Input: part model. Units: mm. Frame: model coordinates. Coordinates: 2 decimals unless noted, no trailing zeros. Write each loop counter-clockwise with the first axis right and the second up, starting at its lowest first coordinate (ties: lowest second). Pieces come first, ordered by that corner, then holes.
from build123d import *

# Parameters (mm, degrees)
F0_W     = 7.9375
F0_H     = 12.7
F0_W_2   = 34.925
F1_DEPTH = 12.7
F3_D     = 4.7625
F5_DEPTH = 50.8


with BuildPart() as f1:
    # F0 (on Front) → F1 (new body, symmetric)
    with BuildSketch(Plane.XZ):
        with Locations((3.96875, -6.35)):
            Rectangle(F0_W, F0_H)
        with Locations((25.4, -6.35)):
            Rectangle(F0_W_2, F0_H)
        with Locations((46.83125, -6.35)):
            Rectangle(F0_W, F0_H)
        with Locations((3.96875, 6.35)):
            Rectangle(F0_W, F0_H)
        with Locations((25.4, 6.35)):
            Rectangle(F0_W_2, F0_H)
        with Locations((46.83125, 6.35)):
            Rectangle(F0_W, F0_H)
    extrude(amount=F1_DEPTH, both=True)

    # F3 (through all)
    with Locations(Plane.XZ.offset(12.7)):
        with Locations((7.9375, 0), (42.8625, 0)):
            Hole(F3_D / 2)

    # F4 (on face) → F5 (cut)
    with BuildSketch(Plane(origin=(0, 0, 0), x_dir=(0, -1, 0), z_dir=(-1, 0, 0))):
        with BuildLine():
            Line((12.7, -12.7), (12.7, 0))
            ThreePointArc((12.7, 0), (8.9802561211, -8.9802561211), (0, -12.7))
            Line((0, -12.7), (12.7, -12.7))
        make_face()
        with BuildLine():
            Line((-12.7, -12.7), (0, -12.7))
            ThreePointArc((0, -12.7), (-8.9802561211, -8.9802561211), (-12.7, 0))
            Line((-12.7, 0), (-12.7, -12.7))
        make_face()
        with BuildLine():
            ThreePointArc((-12.7, 0), (-8.9802561145, 8.9802561276), (1.86e-08, 12.7))
            Line((1.86e-08, 12.7), (-12.7, 12.7))
            Line((-12.7, 12.7), (-12.7, 0))
        make_face()
        with BuildLine():
            ThreePointArc((1.86e-08, 12.7), (8.9802561276, 8.9802561145), (12.7, 0))
            Line((12.7, 0), (12.7, 12.7))
            Line((12.7, 12.7), (1.86e-08, 12.7))
        make_face()
    extrude(amount=-F5_DEPTH, mode=Mode.SUBTRACT)


solid = f1.part
Item 1: Section query A-A, the plane y = -3. Return loops of the section in (x, z).
Item 2: Pull-direction query (Z, two-part tool) for faces 1 (the face through (50.8, 0, 0)), 2 (the face through (10.316, 0.178, 0.105)); classes: released by +Z, released by -Z, zero draft, split by the parting line, or undercut.
Item 3: Pin query (flat end, axial travel): pin 1 Ø6 at (x, y) = (25, 8.5) entering from +Z; pin 2 Ø5 at (x, z) = (40, -10) entering from -Y; pin 3 Ø3 at (x, z) = (42.86, 0) entering from +Y; pin 4 Ø8 at (x, z) = (37, 6.5) entering from -Y. Return the tip coordinate at first contact, or that it passes through.
Item 4: Section query D-D, the plane y = 9. Return loops of the section in (x, z).
Item 5: Section query B-B, the plane x = 35. Return loops of the section in (y, z).
Item 6: Material intervals for line 1 (X direction, y = -4.5, z = 0); line 2 (X direction, y = -10.5, z = 1.25); line 3 (Z direction, x = 37, y = -0.25), sorted ascending.
Item 7: Section query C-C, the plane z = -8. Return loops of the section in (x, y).
The answers:
1. outline: (0, -12.34) - (50.8, -12.34) - (50.8, 12.34) - (0, 12.34) - close; hole circle Ø4.76 at (7.94, 0); hole circle Ø4.76 at (42.86, 0)
2. face 1: zero draft
2. face 2: undercut
3. pin 1: stops at z = 11.45
3. pin 2: stops at y = -10.25
3. pin 3: passes through
3. pin 4: stops at y = -12.45
4. outline: (0, -8.96) - (50.8, -8.96) - (50.8, 8.96) - (0, 8.96) - close; hole circle Ø4.76 at (7.94, 0); hole circle Ø4.76 at (42.86, 0)
5. outline: circle Ø25.4 at (0, 0)
6. line 1: x = 0 to 5.56, 10.32 to 40.48, 45.24 to 50.8
6. line 2: x = 0 to 5.91, 9.96 to 40.84, 44.89 to 50.8
6. line 3: z = -12.7 to 12.7
7. outline: (0, -9.86) - (50.8, -9.86) - (50.8, 9.86) - (0, 9.86) - close
